Autodesk Fusion 360 part; units mm, degrees
sketch "Esquisse1" plane through (0, 0, 0) normal (0, 1, 0) x (1, 0, 0)
  circle A0 centre (0, 0) radius 35
  dimension "d1" = 70
sketch "Esquisse2" plane through (0, 0, 0) normal (0, 1, 0) x (1, 0, 0)
  circle A0 centre (0, 0) radius 32.5
  circle A1 centre (0, 0) radius 35
  dimension "d2" = 65
  dimension "d3" = 70
sketch "Esquisse3" plane through (0, 0, 35.4) normal (0, 0, 1) x (1, 0, 0)
  circle A0 centre (0, 5.75) radius 5.75
  circle A1 centre (0, 5.75) radius 5.75 construction
  circle A2 centre (0, 5.75) radius 3.5
  circle A3 centre (0, 5.75) radius 3
  dimension "d6" = 7
  dimension "d7" = 6
extrude "Extrusion2" add sketch "Esquisse3" along normal blind 2 contours A2 makes body 1
sketch "Esquisse4" plane through (0, 0, 37.4) normal (0, 0, 1) x (1, 0, 0)
  circle A0 centre (0, 5.75) radius 3
  circle A1 centre (0, 5.75) radius 3.5
  line L0 (0, 5.75) -> (0, 23.6) construction
  line L1 (0, 5.75) -> (0, -12.1) construction
  line L2 (0, 23.6) -> (6, 23.6) construction
  line L3 (0, 23.6) -> (-6, 23.6) construction
  line L4 (0, 5.75) -> (-2.5, 5.75)
  line L5 (-2.5, 5.75) -> (-2.5, 23.6)
  line L6 (-2.5, 23.6) -> (0, 23.6)
  line L7 (0, 23.6) -> (0, 5.75)
  line L8 (0, 5.75) -> (2.5, 5.75)
  line L9 (0, 23.6) -> (0, 5.75)
  line L10 (2.5, 5.75) -> (2.5, 23.6)
  line L11 (2.5, 23.6) -> (0, 23.6)
  line L12 (-2.5, 5.75) -> (-2.5, -12.1)
  line L13 (-2.5, -12.1) -> (0, -12.1)
  line L14 (2.5, -12.1) -> (0, -12.1)
  line L15 (2.5, 5.75) -> (2.5, -12.1)
  line L16 (0, 5.75) -> (2.5, 5.75)
  line L17 (0, 5.75) -> (-2.5, 5.75)
  line L18 (0, -12.1) -> (0, 5.75)
  line L19 (0, 5.75) -> (-9.35, 5.75) construction
  line L20 (0, 5.75) -> (9.35, 5.75) construction
  line L21 (-9.35, 5.75) -> (-9.35, 6) construction
  line L22 (-9.35, 6) -> (-9.35, 10) construction
  line L23 (-9.35, 5.75) -> (-9.35, 1.75) construction
  line L24 (9.35, 6) -> (9.35, 10) construction
  line L25 (9.35, 5.75) -> (9.35, 1.75) construction
  line L26 (0, 5.75) -> (-9.35, 5.75)
  line L27 (-9.35, 5.75) -> (-9.35, 3.9)
  line L28 (-9.35, 3.9) -> (0, 3.9)
  line L29 (0, 3.9) -> (0, 5.75)
  line L30 (-9.35, 7.6) -> (0, 7.6)
  line L31 (-9.35, 5.75) -> (-9.35, 7.6)
  line L32 (9.35, 7.6) -> (0, 7.6)
  line L33 (9.35, 5.75) -> (9.35, 7.6)
  line L34 (9.35, 5.75) -> (9.35, 3.9)
  line L35 (9.35, 3.9) -> (0, 3.9)
  line L36 (0, 5.75) -> (9.35, 5.75)
  dimension "d10" = 17.85
  dimension "d11" = 17.85
  dimension "d12" = 2.5
  dimension "d13" = 9.35
  dimension "d14" = 9.35
  dimension "d15" = 4
  dimension "d16" = 1.85
extrude "Extrusion3" add sketch "Esquisse4" along normal blind 2 bodies 1
fillet "Congé1" radius 2.5 4 edges at (-2.5, 23.6, 38.4) (2.5, 23.6, 38.4) (-2.5, -12.1, 38.4) (2.5, -12.1, 38.4) on bodies 1
fillet "Congé2" radius 1.85 4 edges at (-9.35, 7.6, 38.4) (-9.35, 3.9, 38.4) (9.35, 7.6, 38.4) (9.35, 3.9, 38.4) on bodies 1
sketch "Esquisse6" plane through (0, 0, 39.4) normal (0, 0, 1) x (1, 0, 0)
  arc A0 (7.5, 3.9) -> (7.5, 7.6) centre (7.5, 5.75) ccw
  line L0 (7.5, 7.6) -> (2.9711, 7.6)
  arc A1 (2.9711, 7.6) -> (2.5, 8.1995) centre (0, 5.75) ccw
  line L1 (2.5, 8.1995) -> (2.5, 21.1)
  arc A2 (2.5, 21.1) -> (-2.5, 21.1) centre (0, 21.1) ccw
  line L2 (-2.5, 21.1) -> (-2.5, 8.1995)
  arc A3 (-2.5, 8.1995) -> (-2.9711, 7.6) centre (0, 5.75) ccw
  line L3 (-2.9711, 7.6) -> (-7.5, 7.6)
  arc A4 (-7.5, 7.6) -> (-7.5, 3.9) centre (-7.5, 5.75) ccw
  line L4 (-7.5, 3.9) -> (-2.9711, 3.9)
  arc A5 (-2.9711, 3.9) -> (-2.5, 3.3005) centre (0, 5.75) ccw
  line L5 (-2.5, 3.3005) -> (-2.5, -9.6)
  arc A6 (-2.5, -9.6) -> (2.5, -9.6) centre (0, -9.6) ccw
  line L6 (2.5, -9.6) -> (2.5, 3.3005)
  arc A7 (2.5, 3.3005) -> (2.9711, 3.9) centre (0, 5.75) ccw
  line L7 (2.9711, 3.9) -> (7.5, 3.9)
  circle A8 centre (0, 5.75) radius 2
  dimension "d23" = 4
extrude "Extrusion4" cut sketch "Esquisse6" against normal blind 1 contours A8 bodies 1
copy_body "Corps->Comp1" bodies 1 removing the originals makes body 2 in component "servo_arm"
component "servo_arm" placed x (1, 0, 0) y (0, 1, 0) z (0, 0, 1) at (0, 0, 0)
equation "d10 = ( 35.7 / 2 ) * 1 mm"
equation "d11 = ( 35.7 / 2 ) * 1 mm"
equation "d13 = ( 18.7 / 2 ) * 1 mm"
equation "d14 = ( 18.7 / 2 ) * 1 mm"
equation "d16 = ( 3.7 / 2 ) * 1 mm"
Model file for the job. Use its own axes, mm. A direction names the side the tool comes from. Round coordinates to 2 decimals unless told otherwise and drop trailing zeros. Order: outer loops, then holes, each group sorted by start corner. A loop starts at its lowest first (then second) coordinate and runs counter-clockwise, first axis right, second up.
(1) Pull direction X, two halves, no side cores. Call faces 6 (the face through (0, 6, 38.4)), 7 (the face through (8.823, 7.044, 38.414)), 8 (the face through (-8.823, 4.456, 38.414)): released by +X, released by -X, zero draft, split by the parting line, or undercut.
(2) 3-axis set-ups, long thin cutter, end or side, ignore diameter. For faces 1 (the face through (-0.26, 7.733, 38.907)), 2 (the face through (-5, 3.9, 38)), 3 (the face through (5, 7.6, 38)), 4 (the face through (2.5, -3, 38)), 5 (the face through (0, 6, 37.4)): which of +Z, -Z, +X, -X, +Y, -Y reach the whole face in a straight line?
(3) Drill centre lines: line 1 (Y direction, x = 0, z = 38.85); line 2 (Y direction, x = 0, z = 36); line 3 (Z direction, x = -1.5, y = 14.5). Where is each one in solid material? Low to high.
(4) Band-saw the part on A-A (x = -7). List the corners of the cut face in (y, z).
(5) Pin check, flat tips, straight feed: pin 1 (8 mm diameter, centred on x = -7.5, y = 18, fed in from -Z); pin 2 (1.5 mm diameter, centred on x = 1, y = -2, fed in from -Z); pin 3 (1 mm diameter, centred on x = 6.5, z = 38.5, fed in from +Y); pin 4 (3.5 mm diameter, centred on x = 0, y = 5.75, fed in from +Z). Stop position of each tip, or through.
(6) Band-saw the part on B-B (y = -7). List the corners of the cut face in (x, z).
(7) Band-saw the part on C-C (z = 37). List the corners of the cut face in (x, y), then the cut area to 3 significant figures.
Verdict:
1. face 6: undercut
1. face 7: released by +X
1. face 8: released by -X
2. face 1: +Z
2. face 2: +Z, -Z, -X, -Y
2. face 3: +Z, -Z, +X, +Y
2. face 4: +Z, -Z, +X, -Y
2. face 5: -Z
3. line 1: y = -12.1 to 3.75, 7.75 to 23.6
3. line 2: y = 2.25 to 2.75, 8.75 to 9.25
3. line 3: z = 37.4 to 39.4
4. outline: (3.9, 37.4) - (7.6, 37.4) - (7.6, 39.4) - (3.9, 39.4) - close
5. pin 1: passes through
5. pin 2: stops at z = 37.4
5. pin 3: stops at y = 7.6
5. pin 4: stops at z = 38.4
6. outline: (-2.5, 37.4) - (2.5, 37.4) - (2.5, 39.4) - (-2.5, 39.4) - close
7. outline: circle Ø7 at (0, 5.75); hole circle Ø6 at (0, 5.75)
7. area: 10.2 mm2
